```python
from build123d import *

# Parameters (mm, degrees)
SKETCH1_W           = 40
SKETCH1_H           = 20
BOSS_EXTRUDE1_DEPTH = 4
SKETCH5_W           = 40
SKETCH5_H           = 4
BOSS_EXTRUDE2_DEPTH = 16
CUT_EXTRUDE3_DEPTH  = 10
CUT_EXTRUDE5_DEPTH  = 10


with BuildPart() as part:
    # Sketch1 → Boss-Extrude1 (new body)
    with BuildSketch(Plane(origin=(0, 0, 0), x_dir=(1, 0, 0), z_dir=(0, 1, 0))):
        with Locations((-29.259259259, 2.888888889)):
            Rectangle(SKETCH1_W, SKETCH1_H)
    extrude(amount=BOSS_EXTRUDE1_DEPTH)

    # Sketch5 → Boss-Extrude2 (add)
    with BuildSketch(Plane(origin=(0, 4, 0), x_dir=(1, 0, 0), z_dir=(0, 1, 0))):
        with Locations((-29.259259259, -5.111111111)):
            Rectangle(SKETCH5_W, SKETCH5_H)
    extrude(amount=BOSS_EXTRUDE2_DEPTH)

    # Sketch7 → Cut-Extrude3 (cut)
    with BuildSketch(Plane(origin=(0, 4, 0), x_dir=(1, 0, 0), z_dir=(0, 1, 0))):
        with BuildLine():
            Line((-15.259259259, 5.588888889), (-43.259259259, 5.588888889))
            ThreePointArc((-43.259259259, 5.588888889), (-45.409259259, 7.738888889), (-43.259259259, 9.888888889))
            Line((-43.259259259, 9.888888889), (-15.259259259, 9.888888889))
            ThreePointArc((-15.259259259, 9.888888889), (-13.109259259, 7.738888889), (-15.259259259, 5.588888889))
        make_face()
    extrude(amount=-CUT_EXTRUDE3_DEPTH, mode=Mode.SUBTRACT)

    # Sketch8 → Cut-Extrude5 (cut)
    with BuildSketch(Plane(origin=(0, 0, 3.111111111), x_dir=(-1, 0, 0), z_dir=(0, 0, -1))):
        with BuildLine():
            Line((15.259259259, 12.15), (43.259259259, 12.15))
            ThreePointArc((43.259259259, 12.15), (45.409259259, 10), (43.259259259, 7.85))
            Line((43.259259259, 7.85), (15.259259259, 7.85))
            ThreePointArc((15.259259259, 7.85), (13.109259259, 10), (15.259259259, 12.15))
        make_face()
    extrude(amount=-CUT_EXTRUDE5_DEPTH, mode=Mode.SUBTRACT)


solid = part.part
```
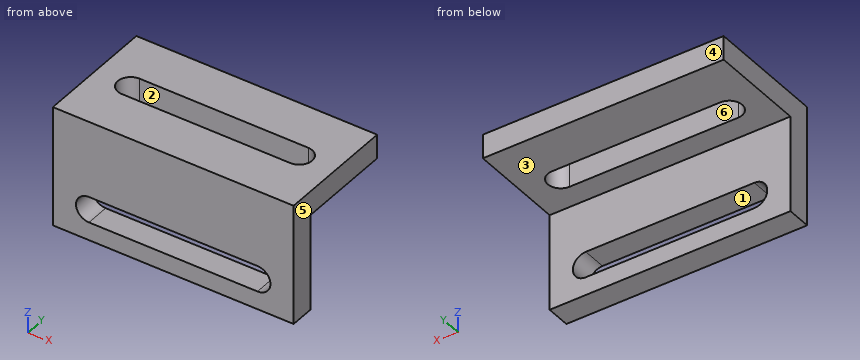
Could you check a few things on this model? Use its own coordinates, in mm. Face numbers are marked on the shaded views. A direction names the side the tool comes from. Give positions to 0.01 mm unless a question says otherwise; leave off trailing zeros. Loops run counter-clockwise (first coordinate to the right, second up) from the corner with the lowest first, then second, coordinate; pieces in that order, holes last. Notation, with made-up numbers: (-6, 69.5) - (4, 69.5) arc R18 cw to (4, 82.5) - close; hole circle Ø6 at (-25.75, 9). An arc over 180 degrees is marked (long way). Use one line per item in the form item = value.
1. I want a section at D-D (z = 5.5). Please give me the cut outline in (x, y).
Response values:
outline = (-49.26, 0) - (-9.26, 0) - (-9.26, 20) - (-49.26, 20) - close; hole (-43.26, 7.85) - (-15.26, 7.85) arc R2.15 ccw to (-15.26, 12.15) - (-43.26, 12.15) arc R2.15 ccw to start
2. On a 3-axis mill with a long thin cutter (end or side, diameter ignored), from which of +Z, -Z, +X, -X, +Y, -Y can I reach the whole of each face in a straight line? I mean the marked faces 1, 2 and 3. Say none if no direction works.
Response values:
face_1 = +Y, -Y
face_2 = +Z, -Z
face_3 = -Z, +X, -X, +Y
3. I need wall thicknesses on probe 1 along Y at (x, z) = (-35, 3.25); probe 2 along Z at (x, y) = (-41.5, 1); probe 3 along Y at (x, z) = (-29, -2). Which ranges of each line are inside material? Lowest first, please.
Response values:
probe_1 = 0 to 7.85, 12.15 to 20
probe_2 = -12.89 to -9.89, -5.59 to 7.11
probe_3 = 0 to 4
4. I want a section at A-A (y = 10). Please give me the cut outline in (x, z), and give its area (3 significant figures).
Response values:
outline = (-49.26, 3.11) - (-45.41, 3.11) - (-45.41, 7.11) - (-49.26, 7.11) - close; (-13.11, 3.11) - (-9.26, 3.11) - (-9.26, 7.11) - (-13.11, 7.11) - close
area = 30.8 mm²
5. I want a section at C-C (y = 2.5). Please give me the cut outline in (x, z), and give its area (3 significant figures).
Response values:
outline = (-49.26, -12.89) - (-9.26, -12.89) - (-9.26, 7.11) - (-49.26, 7.11) - close; hole (-43.26, -9.89) - (-15.26, -9.89) arc R2.15 ccw to (-15.26, -5.59) - (-43.26, -5.59) arc R2.15 ccw to start
area = 665 mm²
6. I want a section at B-B (x = -31.5). Please give me the cut outline in (y, z).
Response values:
outline = (0, -12.89) - (4, -12.89) - (4, -9.89) - (0, -9.89) - close; (0, -5.59) - (4, -5.59) - (4, 3.11) - (7.85, 3.11) - (7.85, 7.11) - (0, 7.11) - close; (12.15, 3.11) - (20, 3.11) - (20, 7.11) - (12.15, 7.11) - close
7. I'm going to push flat-ended pins straight in: pin 1 Ø8 at (x, y) = (-35.5, 12.5) entering from -Z; pin 2 Ø8 at (x, z) = (-36.5, -8.5) entering from +Y; pin 3 Ø3 at (x, z) = (-27, -2.5) entering from -Y. Where does each tip first touch, or does it pass through?
Response values:
pin_1 = 3.11
pin_2 = 4
pin_3 = 0
8. Thinking about a two-plate mould opening in X: for the marked faces 4, 5 and 6, which applies, released by +X, released by -X, zero draft, split by the parting line, or undercut?
Response values:
face_4 = zero draft
face_5 = released by +X
face_6 = undercut
